For this review, take the finished solid that the model builds, in its own axes (mm). Face numbers are marked on the shaded views. A direction names the side the tool comes from. Coordinates: 2 decimals unless noted, no trailing zeros. Write each loop counter-clockwise with the first axis right and the second up, starting at its lowest first coordinate (ties: lowest second). Pieces come first, ordered by that corner, then holes.
```python
from build123d import *

# Parameters (mm, degrees)
SKETCH1_W           = 60
SKETCH1_H           = 15
BOSS_EXTRUDE1_DEPTH = 7
SKETCH2_R           = 2.75
CUT_EXTRUDE1_DEPTH  = 32.705677725
SKETCH3_R           = 5
CUT_EXTRUDE2_DEPTH  = 4
BOSS_EXTRUDE2_DEPTH = 15
SKETCH5_R           = 7.95
CUT_EXTRUDE3_DEPTH  = 42.243181255
FILLET2_R           = 7.5


with BuildPart() as part:
    # Sketch1 → Boss-Extrude1 (new body)
    with BuildSketch(Plane(origin=(0, 0, 0), x_dir=(1, 0, 0), z_dir=(0, 1, 0))):
        Rectangle(SKETCH1_W, SKETCH1_H)
    extrude(amount=BOSS_EXTRUDE1_DEPTH)

    # Sketch2 → Cut-Extrude1 (cut, through all)
    with BuildSketch(Plane(origin=(0, 7, 0), x_dir=(1, 0, 0), z_dir=(0, 1, 0))):
        with Locations(Location((-22.5, 0, 0), (0, 0, 270))):
            Circle(SKETCH2_R)
        with Locations(Location((22.5, 0, 0), (0, 0, 90))):
            Circle(SKETCH2_R)
    extrude(amount=-CUT_EXTRUDE1_DEPTH, mode=Mode.SUBTRACT)

    # Sketch3 → Cut-Extrude2 (cut)
    with BuildSketch(Plane(origin=(0, 7, 0), x_dir=(1, 0, 0), z_dir=(0, 1, 0))):
        with Locations(Location((-22.5, 0, 0), (0, 0, 270))):
            Circle(SKETCH3_R)
        with Locations(Location((22.5, 0, 0), (0, 0, 270))):
            Circle(SKETCH3_R)
    extrude(amount=-CUT_EXTRUDE2_DEPTH, mode=Mode.SUBTRACT)

    # Sketch4 → Boss-Extrude2 (add)
    with BuildSketch(Plane.XY.offset(7.5)):
        with BuildLine():
            Line((-17, 7), (17, 7))
            ThreePointArc((17, 7), (13.464466094, 8.464466094), (12, 12))
            ThreePointArc((12, 12), (0, 24), (-12, 12))
            ThreePointArc((-12, 12), (-13.464466094, 8.464466094), (-17, 7))
        make_face()
    extrude(amount=-BOSS_EXTRUDE2_DEPTH)

    # Sketch5 → Cut-Extrude3 (cut, through all)
    with BuildSketch(Plane.XY.offset(7.5)):
        with Locations((0, 12)):
            Circle(SKETCH5_R)
    extrude(amount=-CUT_EXTRUDE3_DEPTH, mode=Mode.SUBTRACT)

    # Fillet2
    fillet2_edges = [part.edges().sort_by_distance(p)[0] for p in [
        (30, 3.5, 7.5),
        (30, 3.5, -7.5),
        (-30, 3.5, -7.5),
        (-30, 3.5, 7.5),
    ]]
    fillet(fillet2_edges, radius=FILLET2_R - 0.0001)  # a hair under: the kernel refuses the full size


solid = part.part
```
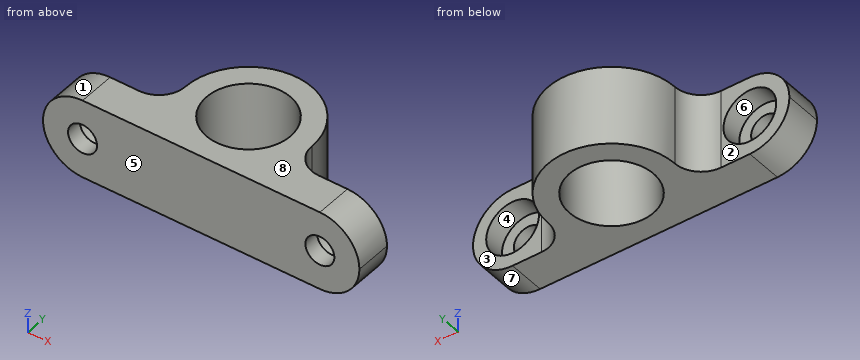
1) Tool access review of the marked faces 1, 2, 3, 4 and 5: name each direction out of +Z, -Z, +X, -X, +Y, -Y from which nothing blocks a thin tool from reaching the whole face with its end or side.
2) Consider section D-D (z = -1). Give the boundary of the cut face in (x, y).
3) Consider section A-A (z = 1.5). Give the boundary of the cut face in (x, y), then the cut area to 3 significant figures.
4) The part is to be moulded in two halves that separate along X. For the marked faces 6, 7 and 8, say which applies: pulls with the +X half, pulls with the -X half, needs draft (parallel to the pull), parting line crosses it, or undercut.
5) Consider section C-C (x = 21.5). Give the boundary of the cut face in (y, z).
6) For L1, parallel to Y at x = 0, z = -2; L2, parallel to X at y = 6.1, z = 0; L3, parallel to X at y = 5.1, z = 0, list the stretches that pass through material, from the lowest coordinate up.
7) Consider section B-B (y = 15.75). Give the boundary of the cut face in (x, z), then the cut area to 3 significant figures.
8) Clearance check with flat-ended pins moving along their axes: P1, Ø1, axis at x = -16.5, z = -1.5, coming from the +Y side; P2, Ø4, axis at x = 26, z = 0.5, coming from the +Y side; P3, Ø4, axis at y = 20.5, z = 4, coming from the +X side. State where each tip first meets the part, or that it passes through.
Results:
1. face 1: +Z, -X, +Y, -Y
1. face 2: +Z, -Z, -X, +Y
1. face 3: +Z, -Z, +X, +Y
1. face 4: +Y
1. face 5: +Z, -Z, +X, -X, -Y
2. outline: (-29.93, 0) - (-25.06, 0) - (-25.06, 3) - (-27.4, 3) - (-27.4, 7) - (-29.93, 7) - close; (-19.94, 0) - (19.94, 0) - (19.94, 3) - (17.6, 3) - (17.6, 7) - (17, 7) arc R5 cw to (12, 12) arc R12 ccw to (-12, 12) arc R5 cw to (-17, 7) - (-17.6, 7) - (-17.6, 3) - (-19.94, 3) - close; (25.06, 0) - (29.93, 0) - (29.93, 7) - (27.4, 7) - (27.4, 3) - (25.06, 3) - close; hole circle Ø15.9 at (0, 12)
3. outline: (-29.85, 0) - (-24.8, 0) - (-24.8, 3) - (-27.27, 3) - (-27.27, 7) - (-29.85, 7) - close; (-20.2, 0) - (20.2, 0) - (20.2, 3) - (17.73, 3) - (17.73, 7) - (17, 7) arc R5 cw to (12, 12) arc R12 ccw to (-12, 12) arc R5 cw to (-17, 7) - (-17.73, 7) - (-17.73, 3) - (-20.2, 3) - close; (24.8, 0) - (29.85, 0) - (29.85, 7) - (27.27, 7) - (27.27, 3) - (24.8, 3) - close; hole circle Ø15.9 at (0, 12)
3. area: 472 mm2
4. face 6: undercut
4. face 7: pulls with the +X half
4. face 8: needs draft
5. outline: (0, -7.5) - (7, -7.5) - (7, -4.9) - (3, -4.9) - (3, -2.56) - (0, -2.56) - close; (0, 2.56) - (3, 2.56) - (3, 4.9) - (7, 4.9) - (7, 7.5) - (0, 7.5) - close
6. L1: y = 0 to 4.05, 19.95 to 24
6. L2: x = -30 to -27.5, -17.5 to -5.33, 5.33 to 17.5, 27.5 to 30
6. L3: x = -30 to -27.5, -17.5 to -3.95, 3.95 to 17.5, 27.5 to 30
7. outline: (-11.4, -7.5) - (-7.01, -7.5) - (-7.01, 7.5) - (-11.4, 7.5) - close; (7.01, -7.5) - (11.4, -7.5) - (11.4, 7.5) - (7.01, 7.5) - close
7. area: 132 mm2
8. P1: stops at y = 7.1
8. P2: stops at y = 7
8. P3: stops at x = 10.09
